The listing builds one solid part. Answer for the finished solid, in the listing's coordinates (mm). A direction names the side the tool comes from. Round coordinates to 2 decimals unless told otherwise and drop trailing zeros. Order: outer loops, then holes, each group sorted by start corner. A loop starts at its lowest first (then second) coordinate and runs counter-clockwise, first axis right, second up. Notation, with made-up numbers: (-7.75, 34.25) - (1.25, 34.25) arc R19 cw to (1.25, 62.25) - close; hole circle Ø2 at (81.25, -31.5). An arc over 180 degrees is marked (long way). One line per item, written item: value. Start each with the question number.
1. Section A-A, the plane z = 5 is taken. Give the vertices of the cut face in (x, y).
2. A tool of negligible diameter and unlimited length cuts with its end or side. For faces 1 (the cylindrical face through (229.986, 254.703, 9.126)), 2 (the flat face through (199, 35, 9)), 3 (the flat face through (196, 144, 0)), from which of +Z, -Z, +X, -X, +Y, -Y can it reach the whole face along a straight path? Write none if from no direction.
3. For a pull along X with two mould halves and no side action, classify faces 4 (the flat face through (315, 0, 9)), 5 (the flat face through (0, 140, 9)), 6 (the cylindrical face through (230.297, 28.986, 9.126)), 7 (the flat face through (397, 140, 9)) as released by +X, released by -X, zero draft, split by the parting line, or undercut.
4. A flat-ended cylindrical pin translates along its axis: P1, Ø2.5, axis at x = 377, y = 162, coming from the +Z side. Find the tip coordinate at first contact, or state that the pin passes through.
5. Straight lines are drawn through the part: line 1 (Y direction, x = 377, z = 9.25); line 2 (X direction, y = 162, z = 7.25); line 3 (X direction, y = 13.5, z = 14). For each, find the intervals that lie inside material, in ascending order.
from build123d import *

# Parameters (mm, degrees)
SKETCH1_W           = 397
SKETCH1_H           = 284
BOSS_EXTRUDE1_DEPTH = 18
SKETCH2_R           = 2
CUT_EXTRUDE1_DEPTH  = 19


with BuildPart() as part:
    # Sketch1 → Boss-Extrude1 (new body)
    with BuildSketch(Plane.XY):
        with Locations((198.5, 142)):
            Rectangle(SKETCH1_W, SKETCH1_H)
    extrude(amount=BOSS_EXTRUDE1_DEPTH)

    # Sketch2 → Cut-Extrude1 (cut, through all)
    with BuildSketch(Plane.XY.offset(18)):
        with Locations((20, 162)):
            Circle(SKETCH2_R)
        with Locations((20, 122)):
            Circle(SKETCH2_R)
        with Locations((377, 122)):
            Circle(SKETCH2_R)
        with Locations((377, 162)):
            Circle(SKETCH2_R)
        with BuildLine():
            Line((236, 284), (161, 284))
            Line((161, 284), (161, 269))
            ThreePointArc((161, 269), (166.857864376, 254.857864376), (181, 249))
            Line((181, 249), (216, 249))
            ThreePointArc((216, 249), (230.142135624, 254.857864376), (236, 269))
            Line((236, 269), (236, 284))
        make_face()
        with BuildLine():
            Line((216, 35), (181, 35))
            ThreePointArc((181, 35), (166.857864376, 29.142135624), (161, 15))
            Line((161, 15), (161, 0))
            Line((161, 0), (236, 0))
            Line((236, 0), (236, 15))
            ThreePointArc((236, 15), (230.142135624, 29.142135624), (216, 35))
        make_face()
    extrude(amount=-CUT_EXTRUDE1_DEPTH, mode=Mode.SUBTRACT)


solid = part.part
Answer list:
1. outline: (0, 0) - (161, 0) - (161, 15) arc R20 cw to (181, 35) - (216, 35) arc R20 cw to (236, 15) - (236, 0) - (397, 0) - (397, 284) - (236, 284) - (236, 269) arc R20 cw to (216, 249) - (181, 249) arc R20 cw to (161, 269) - (161, 284) - (0, 284) - close; hole circle Ø4 at (20, 122); hole circle Ø4 at (20, 162); hole circle Ø4 at (377, 122); hole circle Ø4 at (377, 162)
2. face 1: +Z, -Z, +Y
2. face 2: +Z, -Z, -Y
2. face 3: -Z, +X, -X, +Y, -Y
3. face 4: zero draft
3. face 5: released by -X
3. face 6: undercut
3. face 7: released by +X
4. P1: passes through
5. line 1: y = 0 to 120, 124 to 160, 164 to 284
5. line 2: x = 0 to 18, 22 to 375, 379 to 397
5. line 3: x = 0 to 161, 236 to 397
